Source: three-view drawing plus pictorial views. Frame: mm from the lowest corner of the part. Round coordinates to 2 decimals unless told otherwise and drop trailing zeros. Write each loop counter-clockwise with the first axis right and the second up, starting at its lowest first coordinate (ties: lowest second). Pieces come first, ordered by that corner, then holes. Notation, with made-up numbers: M -25,42.25 L 13,42.25 A31 ccw 13,72.25 Z; hole C -33,60 d10. An arc over 180 degrees is marked long. Answer as CSV lines item,"result". Start each with the question number.
Q1. Section query C-C on z = 0.7. Output: boundary loops of the cut face in (x, y).
Q2. Section query B-B on y = 48. Output: boundary loops of the cut face in (x, z).
Q3. First-contact query: pin 1 (14.5 mm diameter, centred on x = 42, y = 37, fed in from +Z). Flat tip, straight axial feed; report the tip coordinate or a pass-through.
Q4. Ray query, probe 1 along Y at (x, z) = (45.5, 1.05); probe 2 along X at (y, z) = (19.5, 3.5); probe 3 along Y at (x, z) = (27.5, 2.9). Return the intervals inside material, ascending.
Q5. Section query A-A on x = 45. Output: boundary loops of the cut face in (y, z).
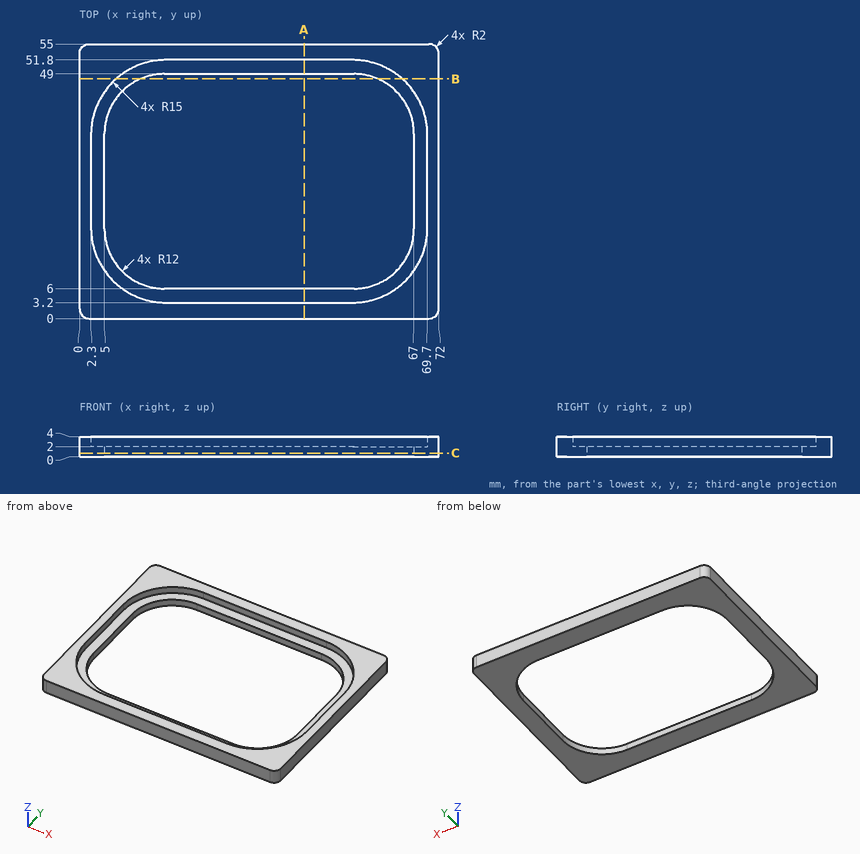
Entries:
1,outline,"M 0,2 A2 ccw 2,0 L 70,0 A2 ccw 72,2 L 72,53 A2 ccw 70,55 L 2,55 A2 ccw 0,53 Z; hole M 5,18 A12 ccw 17,6 L 55,6 A12 ccw 67,18 L 67,37 A12 ccw 55,49 L 17,49 A12 ccw 5,37 Z"
2,outline,"M 0,0 L 12.2,0 L 12.2,2 L 7.32,2 L 7.32,4 L 0,4 Z; M 59.8,0 L 72,0 L 72,4 L 64.68,4 L 64.68,2 L 59.8,2 Z"
3,pin 1,"passes through"
4,probe 1,"y = 0 to 6, 49 to 55"
4,probe 2,"x = 0 to 2.3, 69.7 to 72"
4,probe 3,"y = 0 to 3.2, 51.8 to 55"
5,outline,"M 0,0 L 6,0 L 6,2 L 3.2,2 L 3.2,4 L 0,4 Z; M 49,0 L 55,0 L 55,4 L 51.8,4 L 51.8,2 L 49,2 Z"
